The listing builds one solid part. Answer for the finished solid, in the listing's coordinates (mm). Face numbers are marked on the shaded views. Round coordinates to 2 decimals unless told otherwise and drop trailing zeros. Write each loop counter-clockwise with the first axis right and the second up, starting at its lowest first coordinate (ties: lowest second). Pieces come first, ordered by that corner, then holes.
Item 1: Find the intervals of material crossed by probe 1 along X at (y, z) = (1.8, 0); probe 2 along Z at (x, y) = (-13.5, 5); probe 3 along Z at (x, y) = (21, 7), in increasing order.
Item 2: Find section B-B on x = 0. Give the vertices of the cut face in (y, z), then the cut area to 4 significant figures.
Item 3: Find section C-C on y = 6.75. Give the vertices of the cut face in (x, z).
Item 4: Find section A-A on z = 0. Give the vertices of the cut face in (x, y), then the cut area to 3 significant figures.
Item 5: This flat-tipped pin is pushed along its axis until it touches: pin 1 (5 mm diameter, centred on x = -26.5, z = 3, fed in from +Y). Where does it stop, or does it pass through?
Item 6: For a pull along Z with two mould halves and no side action, classify the marked faces 1, 2, 3 and 4 as +Z half, -Z half, draft (parallel to the pull), parting line (faces both ways), or undercut.
Item 7: Find section D-D on z = 21. Give the vertices of the cut face in (x, y).
```python
from build123d import *

# Parameters (mm, degrees)
SKETCH1_W           = 66.8
SKETCH1_H           = 54.8
BOSS_EXTRUDE1_DEPTH = 6
CHAMFER2_SIZE       = 0.5
FILLET2_R           = 2
SHELL3_T            = -2.4
BOSS_EXTRUDE4_DEPTH = 3.4
CUT_EXTRUDE2_REACH  = 46.212
SKETCH6_R           = 12.5


with BuildPart() as part:
    # Sketch1 → Boss-Extrude1 (new body)
    with BuildSketch(Plane(origin=(0, 0, 0), x_dir=(1, 0, 0), z_dir=(0, 1, 0))):
        Rectangle(SKETCH1_W, SKETCH1_H)
    extrude(amount=BOSS_EXTRUDE1_DEPTH)

    # Chamfer2
    chamfer2_edges = [part.edges().sort_by_distance(p)[0] for p in [
        (0, 0, 27.4),
        (-33.4, 0, 0),
        (0, 0, -27.4),
        (33.4, 0, 0),
    ]]
    chamfer(chamfer2_edges, length=CHAMFER2_SIZE)

    # Fillet2
    # the kernel refuses this fillet: 2 mm, written as the material it takes off along each edge
    with BuildSketch(Plane(origin=(33.4, -4.5, 27.4), x_dir=(0, 0, -1), z_dir=(0, 1, 0)), Plane(origin=(33.4, -4.5, -27.4), x_dir=(-1, 0, 0), z_dir=(0, 1, 0))) as fillet2_piece_1:
        with BuildLine():
            CenterArc((FILLET2_R, FILLET2_R), FILLET2_R, 180, 90)
            Line((0, FILLET2_R), (0, 0))
            Line((0, 0), (FILLET2_R, 0))
        make_face()
    extrude(amount=15.5, mode=Mode.SUBTRACT)
    with BuildSketch(Plane(origin=(-33.4, -4.5, 27.4), x_dir=(0, 0, -1), z_dir=(0, 1, 0)), Plane(origin=(-33.4, -4.5, -27.4), x_dir=(1, 0, 0), z_dir=(0, 1, 0))) as fillet2_piece_2:
        with BuildLine():
            CenterArc((FILLET2_R, -FILLET2_R), FILLET2_R, 90, 90)
            Line((0, -FILLET2_R), (0, 0))
            Line((0, 0), (FILLET2_R, 0))
        make_face()
    extrude(amount=15.5, mode=Mode.SUBTRACT)

    # Shell3
    shell3_openings = [part.faces().sort_by_distance(p)[0] for p in [
        (0, 6, 0),
    ]]
    offset(amount=SHELL3_T, openings=shell3_openings, kind=Kind.INTERSECTION)

    # Sketch5 → Boss-Extrude4 (add)
    with BuildSketch(Plane(origin=(0, 6, 0), x_dir=(1, 0, 0), z_dir=(0, 1, 0))):
        with BuildLine():
            Line((33.4, -25.4), (33.4, 25.4))
            ThreePointArc((33.4, 25.4), (32.814213562, 26.814213562), (31.4, 27.4))
            Line((31.4, 27.4), (-31.4, 27.4))
            ThreePointArc((-31.4, 27.4), (-32.814213562, 26.814213562), (-33.4, 25.4))
            Line((-33.4, 25.4), (-33.4, -25.4))
            ThreePointArc((-33.4, -25.4), (-32.814213562, -26.814213562), (-31.4, -27.4))
            Line((-31.4, -27.4), (31.4, -27.4))
            ThreePointArc((31.4, -27.4), (32.814213562, -26.814213562), (33.4, -25.4))
        make_face()
        with BuildLine():
            Line((-31.4, -26.15), (31.4, -26.15))
            ThreePointArc((31.4, -26.15), (31.930330086, -25.930330086), (32.15, -25.4))
            Line((32.15, -25.4), (32.15, 25.4))
            ThreePointArc((32.15, 25.4), (31.930330086, 25.930330086), (31.4, 26.15))
            Line((31.4, 26.15), (-31.4, 26.15))
            ThreePointArc((-31.4, 26.15), (-31.930330086, 25.930330086), (-32.15, 25.4))
            Line((-32.15, 25.4), (-32.15, -25.4))
            ThreePointArc((-32.15, -25.4), (-31.930330086, -25.930330086), (-31.4, -26.15))
        make_face(mode=Mode.SUBTRACT)
    extrude(amount=BOSS_EXTRUDE4_DEPTH)

    # Sketch6 → Cut-Extrude2 (cut, up to next)
    with BuildSketch(Plane.XZ, mode=Mode.PRIVATE) as cut_extrude2_sk1:
        with Locations(Location((0, 0, 0), (0, 0, 270))):
            Circle(SKETCH6_R)
    cut_extrude2_tool1 = extrude(cut_extrude2_sk1.sketch, amount=-CUT_EXTRUDE2_REACH, mode=Mode.PRIVATE) & part.part
    add(cut_extrude2_tool1.solids().sort_by_distance((0, 0, 0))[0], mode=Mode.SUBTRACT)


solid = part.part
```
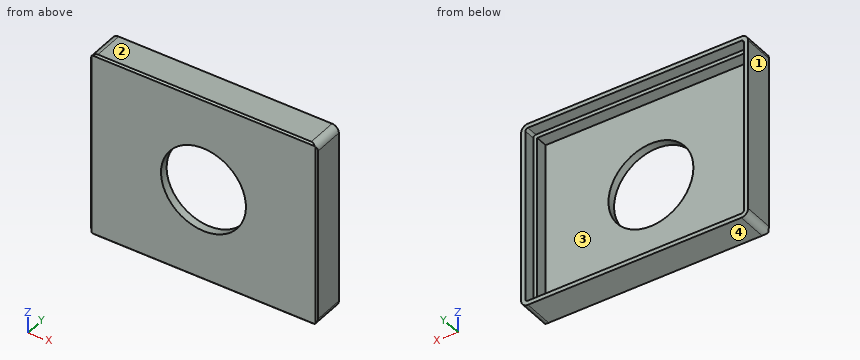
Check values:
1. probe 1: x = -33.4 to -12.5, 12.5 to 33.4
1. probe 2: z = -27.4 to -25, 25 to 27.4
1. probe 3: z = -27.4 to -26.15, 26.15 to 27.4
2. outline: (0, -26.9) - (0.5, -27.4) - (9.4, -27.4) - (9.4, -26.15) - (6, -26.15) - (6, -25) - (2.4, -25) - (2.4, -12.5) - (0, -12.5) - close; (0, 12.5) - (2.4, 12.5) - (2.4, 25) - (6, 25) - (6, 26.15) - (9.4, 26.15) - (9.4, 27.4) - (0.5, 27.4) - (0, 26.9) - close
2. area: 97.05 mm2
3. outline: (-33.4, -25.4) arc R2 ccw to (-31.4, -27.4) - (31.4, -27.4) arc R2 ccw to (33.4, -25.4) - (33.4, 25.4) arc R2 ccw to (31.4, 27.4) - (-31.4, 27.4) arc R2 ccw to (-33.4, 25.4) - close; hole (-32.15, -25.4) arc R0.75 ccw to (-31.4, -26.15) - (31.4, -26.15) arc R0.75 ccw to (32.15, -25.4) - (32.15, 25.4) arc R0.75 ccw to (31.4, 26.15) - (-31.4, 26.15) arc R0.75 ccw to (-32.15, 25.4) - close
4. outline: (-33.4, 0.5) - (-32.9, 0) - (-12.5, 0) - (-12.5, 2.4) - (-31, 2.4) - (-31, 6) - (-32.15, 6) - (-32.15, 9.4) - (-33.4, 9.4) - close; (12.5, 0) - (32.9, 0) - (33.4, 0.5) - (33.4, 9.4) - (32.15, 9.4) - (32.15, 6) - (31, 6) - (31, 2.4) - (12.5, 2.4) - close
4. area: 126 mm2
5. pin 1: stops at y = 2.4
6. face 1: draft
6. face 2: +Z half
6. face 3: undercut
6. face 4: -Z half
7. outline: (-33.4, 0.5) - (-32.9, 0) - (32.9, 0) - (33.4, 0.5) - (33.4, 9.4) - (32.15, 9.4) - (32.15, 6) - (31, 6) - (31, 2.4) - (-31, 2.4) - (-31, 6) - (-32.15, 6) - (-32.15, 9.4) - (-33.4, 9.4) - close
